from build123d import *

# Parameters (mm, degrees)
F0_R     = 11.25
F1_DEPTH = 4
F2_R     = 4.5
F3_DEPTH = 6
F6_R     = 2
F7_DEPTH = 4


with BuildPart() as f1:
    # F0 (on Top) → F1 (new body)
    with BuildSketch(Plane.XY):
        Circle(F0_R)
    extrude(amount=F1_DEPTH)

    # F2 (on face) → F3 (join)
    with BuildSketch(Plane.XY.offset(4)):
        Circle(F2_R)
    extrude(amount=F3_DEPTH)

    # F4 (on Front) → F5 (revolve)
    with BuildSketch(Plane.XZ):
        with BuildLine():
            Line((20.5, 16), (0, 16))
            Line((0, 16), (0, 10))
            Line((0, 10), (4.5, 10))
            Line((4.5, 10), (26.5, 17))
            ThreePointArc((26.5, 17), (25.5, 18), (24.5, 17))
            Line((24.5, 17), (20.5, 16))
        make_face()
    revolve(axis=Axis((0, 0, 19.201497), (0, 0, 1)))

    # F6 (on face) → F7 (cut, through all)
    with BuildSketch(Plane(origin=(0, 0, 0), x_dir=(1, 0, 0), z_dir=(0, 0, -1))):
        with Locations((-5.629165, -3.25)):
            Circle(F6_R)
        with Locations((5.629165, -3.25)):
            Circle(F6_R)
        with Locations((0, 6.5)):
            Circle(F6_R)
    extrude(amount=-F7_DEPTH, mode=Mode.SUBTRACT)


solid = f1.part
Could you check a few things on this model? Use its own coordinates, in mm. A direction names the side the tool comes from. Coordinates: 2 decimals unless noted, no trailing zeros. Order: outer loops, then holes, each group sorted by start corner. A loop starts at its lowest first (then second) coordinate and runs counter-clockwise, first axis right, second up. Notation, with made-up numbers: (-24, -11) - (19, -11) arc R20 ccw to (19, 1) - close; hole circle Ø6 at (60, -26). An arc over 180 degrees is marked (long way). Answer in a Markdown table with one row per item. Add a question column.
(1) If we section it at C-C, the plane z = 13.5: Please give me the cut outline in (x, y), then the cut area to 3 significant figures.
(2) If we section it at B-B, the plane z = 1.5: Please give me the cut outline in (x, y), then the cut area to 3 significant figures.
(3) If we section it at A-A, the plane y = 0: Please give me the cut outline in (x, z), then the cut area to 3 significant figures.
(4) On a 3-axis mill with a long thin cutter (end or side, diameter ignored), from which of +Z, -Z, +X, -X, +Y, -Y can I reach the whole of each face in a straight line? I mean faces 1 (the face through (-0.59, 4.46, 6.96)), 2 (the face through (0, 0, 0)), 3 (the face through (0, 0, 16)), 4 (the face through (4.042, 4.467, 1.972)). Say none if no direction works.
(5) Will these pins go through, and if not, where does the flat tip stop? pin 1 (10 mm diameter, centred on y = -5, z = 4.5, fed in from +X); pin 2 (5 mm diameter, centred on x = 1.5, z = 15.5, fed in from +Y); pin 3 (2.5 mm diameter, centred on x = 0, y = -6.5, fed in from -Z).
(6) If we section it at D-D, the plane y = -6.5: State how many separate pieces and enclosed holes the cut face has, then the cut area to 3 significant figures.
(7) If we mould it in two halves opening along X, with no side actions, what happens to faces 5 (the face through (19.74, 6.22, 16.05)), 6 (the face through (5.19, -9.98, 1.97)), 7 (the face through (5, 0, 4))? For each: released by +X, released by -X, zero draft, split by the parting line, or undercut.
(8) I need wall thicknesses on L1, parallel to X at y = 3.25, z = 2.2; L2, parallel to X at y = -6.5, z = 2.95; L3, parallel to Z at x = 3, y = 8. Which ranges of each line are inside material? Lowest first, please.
Results are:
| question | item | result |
|---|---|---|
| 1 | outline | circle Ø31 at (0, 0) |
| 1 | area | 755 mm2 |
| 2 | outline | circle Ø22.5 at (0, 0); hole circle Ø4 at (-5.63, 3.25); hole circle Ø4 at (0, -6.5); hole circle Ø4 at (5.63, 3.25) |
| 2 | area | 360 mm2 |
| 3 | outline | (-26.5, 17) - (-4.5, 10) - (-4.5, 4) - (-11.25, 4) - (-11.25, 0) - (11.25, 0) - (11.25, 4) - (4.5, 4) - (4.5, 10) - (26.5, 17) arc R1 ccw to (24.5, 17) - (20.5, 16) - (-20.5, 16) - (-24.5, 17) arc R1 ccw to start |
| 3 | area | 319 mm2 |
| 4 | face 1 | none |
| 4 | face 2 | -Z, +X, -X, +Y, -Y |
| 4 | face 3 | +Z |
| 4 | face 4 | -Z |
| 5 | pin 1 | stops at x = 11.25 |
| 5 | pin 2 | stops at y = 26.5 |
| 5 | pin 3 | stops at z = 10.24 |
| 6 | separate pieces | 3 |
| 6 | enclosed holes | 0 |
| 6 | area | 206 mm2 |
| 7 | face 5 | undercut |
| 7 | face 6 | split by the parting line |
| 7 | face 7 | zero draft |
| 8 | L1 | x = -10.77 to -7.63, -3.63 to 3.63, 7.63 to 10.77 |
| 8 | L2 | x = -9.18 to -2, 2 to 9.18 |
| 8 | L3 | z = 0 to 4, 11.29 to 16 |
